from build123d import *

# Parameters (mm, degrees)
SKETCH1_W           = 23
SKETCH1_H           = 65
BOSS_EXTRUDE1_DEPTH = 66
SKETCH2_W           = 60
SKETCH2_H           = 17
CUT_EXTRUDE1_DEPTH  = 66
CUT_EXTRUDE2_REACH  = 25
SKETCH3_W           = 32
SKETCH3_H           = 53
CUT_EXTRUDE3_REACH  = 25
SKETCH5_R           = 4.5
SKETCH5_R_2         = 2.530586218
SKETCH5_R_3         = 2.69284222


with BuildPart() as part:
    # Sketch1 → Boss-Extrude1 (new body)
    with BuildSketch(Plane(origin=(0, 0, 0), x_dir=(0, 0, -1), z_dir=(1, 0, 0))):
        with Locations((-11.5, -32.5)):
            Rectangle(SKETCH1_W, SKETCH1_H)
    extrude(amount=-BOSS_EXTRUDE1_DEPTH)

    # Sketch2 → Cut-Extrude1 (cut, through all)
    with BuildSketch(Plane(origin=(0, 0, 0), x_dir=(1, 0, 0), z_dir=(0, 1, 0))):
        with Locations((-33, -11.5)):
            Rectangle(SKETCH2_W, SKETCH2_H)
    extrude(amount=-CUT_EXTRUDE1_DEPTH, mode=Mode.SUBTRACT)

    # Sketch3 → Cut-Extrude2 (cut, up to next)
    with BuildSketch(Plane.XY.offset(23), mode=Mode.PRIVATE) as cut_extrude2_sk1:
        with Locations((-33, -26.5)):
            Rectangle(SKETCH3_W, SKETCH3_H)
    cut_extrude2_tool1 = extrude(cut_extrude2_sk1.sketch, amount=-CUT_EXTRUDE2_REACH, mode=Mode.PRIVATE) & part.part
    add(cut_extrude2_tool1.solids().sort_by_distance((-33, -26.5, 23))[0], mode=Mode.SUBTRACT)

    # Sketch5 → Cut-Extrude3 (cut, up to next)
    with BuildSketch(Plane(origin=(0, 0, 0), x_dir=(-1, 0, 0), z_dir=(0, 0, -1)), mode=Mode.PRIVATE) as cut_extrude3_sk1:
        with Locations((33, -37)):
            Circle(SKETCH5_R)
    cut_extrude3_tool1 = extrude(cut_extrude3_sk1.sketch, amount=-CUT_EXTRUDE3_REACH, mode=Mode.PRIVATE) & part.part
    add(cut_extrude3_tool1.solids().sort_by_distance((-33, -37, 0))[0], mode=Mode.SUBTRACT)
    # Sketch5 → Cut-Extrude3 (cut, up to next)
    with BuildSketch(Plane(origin=(0, 0, 0), x_dir=(-1, 0, 0), z_dir=(0, 0, -1)), mode=Mode.PRIVATE) as cut_extrude3_sk2:
        with Locations((8, -7)):
            Circle(SKETCH5_R_2)
    cut_extrude3_tool2 = extrude(cut_extrude3_sk2.sketch, amount=-CUT_EXTRUDE3_REACH, mode=Mode.PRIVATE) & part.part
    add(cut_extrude3_tool2.solids().sort_by_distance((-8, -7, 0))[0], mode=Mode.SUBTRACT)
    # Sketch5 → Cut-Extrude3 (cut, up to next)
    with BuildSketch(Plane(origin=(0, 0, 0), x_dir=(-1, 0, 0), z_dir=(0, 0, -1)), mode=Mode.PRIVATE) as cut_extrude3_sk3:
        with Locations((58, -7)):
            Circle(SKETCH5_R_3)
    cut_extrude3_tool3 = extrude(cut_extrude3_sk3.sketch, amount=-CUT_EXTRUDE3_REACH, mode=Mode.PRIVATE) & part.part
    add(cut_extrude3_tool3.solids().sort_by_distance((-58, -7, 0))[0], mode=Mode.SUBTRACT)


solid = part.part
Check sheet for the modelled part. Datum: model origin and axes. Units: mm. A direction names the side the tool comes from. Round coordinates to 2 decimals unless told otherwise and drop trailing zeros. Order: outer loops, then holes, each group sorted by start corner. A loop starts at its lowest first (then second) coordinate and runs counter-clockwise, first axis right, second up.
(1) Cross-section at C-C, the plane y = -37. Enter the section's corners in (x, z), and give its area (3 significant figures).
(2) Cross-section at A-A, the plane x = -8. Enter the section's corners in (y, z), and give its area (3 significant figures).
(3) Draft check along Y on faces 1 (the flat face through (-3, -32, 12)), 2 (the flat face through (-26, 0, 2)), 3 (the cylindrical face through (-5.99, -8.54, 1.48)). Enter one of: pulls with the +Y half, pulls with the -Y half, needs draft (parallel to the pull), parting line crosses it, or undercut.
(4) Go/stop test with a flat-tipped pin: P1, Ø2.5, axis at x = -30.5, z = 21.5, coming from the +Y side. Record where the tip stops, or that it passes through.
(5) Access from +Z, -Z, +X, -X, +Y, -Y to the whole of each face (thin tool, end or side, straight path). Record for faces 4 (the cylindrical face through (-60.5, -8, 1.5)), 5 (the flat face through (-49, -27, 22)), 6 (the flat face through (-66, -32, 12)), 7 (the flat face through (-33, -32, 3)), 8 (the flat face through (-33, -55, 23)).
(6) Cross-section at B-B, the plane x = -50.5. Enter the section's corners in (y, z), and give its area (3 significant figures).
(7) Scan lines: probe 1 along Z at (x, y) = (-9, -33.5); probe 2 along Y at (x, z) = (-33, 1.9); probe 3 along X at (y, z) = (-13.5, 3.75). Record each from-to range of solid material in increasing order.
(8) Cross-section at D-D, the plane z = 14.75. Enter the section's corners in (x, y).
Check sheet entries:
1. outline: (-66, 0) - (-37.5, 0) - (-37.5, 3) - (-63, 3) - (-63, 20) - (-49, 20) - (-49, 23) - (-66, 23) - close; (-28.5, 0) - (0, 0) - (0, 23) - (-17, 23) - (-17, 20) - (-3, 20) - (-3, 3) - (-28.5, 3) - close
1. area: 375 mm2
2. outline: (-65, 0) - (-9.53, 0) - (-9.53, 3) - (-65, 3) - close; (-65, 20) - (0, 20) - (0, 23) - (-65, 23) - close; (-4.47, 0) - (0, 0) - (0, 3) - (-4.47, 3) - close
2. area: 375 mm2
3. face 1: needs draft
3. face 2: pulls with the +Y half
3. face 3: undercut
4. P1: stops at y = -53
5. face 4: -Z
5. face 5: +Z, +Y
5. face 6: +Z, -Z, -X, +Y, -Y
5. face 7: +Y, -Y
5. face 8: +Z, +X, -X, +Y, -Y
6. outline: (-65, 0) - (0, 0) - (0, 3) - (-65, 3) - close; (-65, 20) - (0, 20) - (0, 23) - (-65, 23) - close
6. area: 390 mm2
7. probe 1: z = 0 to 3, 20 to 23
7. probe 2: y = -65 to -41.5, -32.5 to 0
7. probe 3: x = -66 to -63, -3 to 0
8. outline: (-66, -65) - (-63, -65) - (-63, 0) - (-66, 0) - close; (-3, -65) - (0, -65) - (0, 0) - (-3, 0) - close
